Here's how the part is built. I have some questions about the finished solid (model axes, mm). A direction names the side the tool comes from. Give positions to 0.01 mm unless a question says otherwise; leave off trailing zeros. Write each loop counter-clockwise with the first axis right and the second up, starting at its lowest first coordinate (ties: lowest second). Pieces come first, ordered by that corner, then holes. Notation, with made-up numbers: (82, 70.5) - (97, 70.5) arc R19 ccw to (97, 102.5) - close; hole circle Ø8 at (55.5, 85). An arc over 180 degrees is marked (long way). Use a Markdown table: item, result.
```python
from build123d import *

# Parameters (mm, degrees)
BOSS_EXTRUDE1_DEPTH = 304.8
SKETCH3_R           = 6.35
BOSS_EXTRUDE2_DEPTH = 76.2


with BuildPart() as part:
    # Sketch1 → Boss-Extrude1 (new body)
    with BuildSketch(Plane.XY):
        with BuildLine():
            Line((19.05, 31.75), (-19.05, 31.75))
            ThreePointArc((-19.05, 31.75), (-28.030256121, 28.030256121), (-31.75, 19.05))
            Line((-31.75, 19.05), (-31.75, -19.05))
            ThreePointArc((-31.75, -19.05), (-28.030256121, -28.030256121), (-19.05, -31.75))
            Line((-19.05, -31.75), (19.05, -31.75))
            ThreePointArc((19.05, -31.75), (28.030256121, -28.030256121), (31.75, -19.05))
            Line((31.75, -19.05), (31.75, 19.05))
            ThreePointArc((31.75, 19.05), (28.030256121, 28.030256121), (19.05, 31.75))
        make_face()
        with BuildLine():
            ThreePointArc((-25.4, -19.05), (-23.540128061, -23.540128061), (-19.05, -25.4))
            Line((-19.05, -25.4), (19.05, -25.4))
            ThreePointArc((19.05, -25.4), (23.540128061, -23.540128061), (25.4, -19.05))
            Line((25.4, -19.05), (25.4, 19.05))
            ThreePointArc((25.4, 19.05), (23.540128061, 23.540128061), (19.05, 25.4))
            Line((19.05, 25.4), (-19.05, 25.4))
            ThreePointArc((-19.05, 25.4), (-23.540128061, 23.540128061), (-25.4, 19.05))
            Line((-25.4, 19.05), (-25.4, -19.05))
        make_face(mode=Mode.SUBTRACT)
    extrude(amount=BOSS_EXTRUDE1_DEPTH)

    # Sketch3 → Boss-Extrude2 (add, symmetric)
    with BuildSketch(Plane(origin=(0, 0, 0), x_dir=(1, 0, 0), z_dir=(0, 1, 0))):
        with Locations((0, -19.05)):
            Circle(SKETCH3_R)
    extrude(amount=BOSS_EXTRUDE2_DEPTH, both=True)


solid = part.part
```
Item 1: For faces 1 (the cylindrical face through (23.49, -23.59, 150.27)), 2 (the cylindrical face through (-1.38, -53.66, 25.25)), 3 (the cylindrical face through (-1.38, 54.29, 25.25)), which set-ups out of +Z, -Z, +X, -X, +Y, -Y let a thin tool reach every point of the face, with its end or its side?
Values:
| item | result |
|---|---|
| face 1 | +Z, -Z |
| face 2 | -Y |
| face 3 | +Y |
Item 2: If we section it at C-C, the plane z = 19.05: Write out the boundary of the cut face in (x, y).
Values:
| item | result |
|---|---|
| outline | (-31.75, -19.05) arc R12.7 ccw to (-19.05, -31.75) - (-6.35, -31.75) - (-6.35, -76.2) - (6.35, -76.2) - (6.35, -31.75) - (19.05, -31.75) arc R12.7 ccw to (31.75, -19.05) - (31.75, 19.05) arc R12.7 ccw to (19.05, 31.75) - (6.35, 31.75) - (6.35, 76.2) - (-6.35, 76.2) - (-6.35, 31.75) - (-19.05, 31.75) arc R12.7 ccw to (-31.75, 19.05) - close; hole (-25.4, -19.05) arc R6.35 ccw to (-19.05, -25.4) - (-6.35, -25.4) - (-6.35, 25.4) - (-19.05, 25.4) arc R6.35 ccw to (-25.4, 19.05) - close; hole (6.35, -25.4) - (19.05, -25.4) arc R6.35 ccw to (25.4, -19.05) - (25.4, 19.05) arc R6.35 ccw to (19.05, 25.4) - (6.35, 25.4) - close |
Item 3: If we section it at B-B, the plane z = 137: Write out the boundary of the cut face in (x, y), plus the area to 3 significant figures.
Values:
| item | result |
|---|---|
| outline | (-31.75, -19.05) arc R12.7 ccw to (-19.05, -31.75) - (19.05, -31.75) arc R12.7 ccw to (31.75, -19.05) - (31.75, 19.05) arc R12.7 ccw to (19.05, 31.75) - (-19.05, 31.75) arc R12.7 ccw to (-31.75, 19.05) - close; hole (-25.4, -19.05) arc R6.35 ccw to (-19.05, -25.4) - (19.05, -25.4) arc R6.35 ccw to (25.4, -19.05) - (25.4, 19.05) arc R6.35 ccw to (19.05, 25.4) - (-19.05, 25.4) arc R6.35 ccw to (-25.4, 19.05) - close |
| area | 1,350 mm2 |
Item 4: Thinking about a two-plate mould opening in X: for faces 4 (the cylindrical face through (28.13, 27.93, 150.27)), 5 (the cylindrical face through (-28.13, -27.93, 150.27)), 6 (the cylindrical face through (-1.38, 0.36, 25.25)), which applies, +X half, -X half, draft (parallel to the pull), parting line (faces both ways), or undercut?
Values:
| item | result |
|---|---|
| face 4 | +X half |
| face 5 | -X half |
| face 6 | undercut |
Item 5: I need wall thicknesses on line 1 along Y through (x, z) = (-10.5, 224); line 2 along Z through (x, y) = (-0.5, 51). Which ranges of each line are inside material? Lowest first, please. Write a range as [from, to].
Values:
| item | result |
|---|---|
| line 1 | y = [-31.75, -25.4], [25.4, 31.75] |
| line 2 | z = [12.72, 25.38] |
Item 6: If we section it at A-A, the plane x = 10: Write out the boundary of the cut face in (y, z), plus the area to 3 significant figures.
Values:
| item | result |
|---|---|
| outline | (-31.75, 0) - (-25.4, 0) - (-25.4, 304.8) - (-31.75, 304.8) - close; (25.4, 0) - (31.75, 0) - (31.75, 304.8) - (25.4, 304.8) - close |
| area | 3,870 mm2 |
Item 7: Will these pins go through, and if not, where does the flat tip stop? pin 1 Ø10 at (x, z) = (24.5, 205.5) entering from +Y; pin 2 Ø11.5 at (x, z) = (-9.5, 162) entering from +Y; pin 3 Ø3 at (x, z) = (-0.5, 73) entering from -Y; pin 4 Ø6 at (y, z) = (-36, 143) entering from +X.
Values:
| item | result |
|---|---|
| pin 1 | stops at y = 31.74 |
| pin 2 | stops at y = 31.75 |
| pin 3 | stops at y = -31.75 |
| pin 4 | passes through |
Item 8: If we section it at D-D, the plane y = -63: Write out the boundary of the cut face in (x, z).
Values:
| item | result |
|---|---|
| outline | circle Ø12.7 at (0, 19.05) |
